Source: CAD feature listing. Evaluate the final solid. Frame: model axes, mm. A direction names the side the tool comes from. Coordinates: 2 decimals unless noted, no trailing zeros. Order: outer loops, then holes, each group sorted by start corner. A loop starts at its lowest first (then second) coordinate and runs counter-clockwise, first axis right, second up. Notation, with made-up numbers: (40.25, 36) -> (96.25, 36) arc R27 cw to (96.25, 65) -> close; hole circle Ø4 at (49, -34). An arc over 180 degrees is marked (long way). Put each result on its own line as item: value.
from build123d import *

# Parameters (mm, degrees)
EXTRUDE_1_DEPTH                   = 3
SKETCH_2_R                        = 1.5
SKETCH_2_R_2                      = 0.75
EXTRUDE_2_DEPTH                   = 73
SKETCH_3_W                        = 42
SKETCH_3_H                        = 3.5
SKETCH_3_W_2                      = 3.2
SKETCH_3_H_2                      = 20.2
CUT_EXTRUDE_1_DEPTH               = 83.725086884
CUT_EXTRUDE_2_REACH               = 84.028
CUT_EXTRUDE_2_OFFSET_FROM_SURFACE = 1.5
CUT_EXTRUDE_START                 = -1.5
SKETCH_4_W                        = 44.5
SKETCH_4_H                        = 1
SKETCH_4_3_W                      = 22
SKETCH_4_3_H                      = 1
CUT_EXTRUDE_3_DEPTH               = 37.5
SKETCH_5_W                        = 3
SKETCH_5_H                        = 1
EXTRUDE_3_DEPTH                   = 34.5
SKETCH_6_R                        = 0.35
CUT_EXTRUDE_4_DEPTH               = 80.653562381
SKETCH_7_W                        = 24.036657481
SKETCH_7_H                        = 1
CUT_EXTRUDE_5_DEPTH               = 1.5
CUT_EXTRUDE_6_DEPTH               = 80.653562381


with BuildPart() as part:
    # 草图1 → 凸台-拉伸1 (new body)
    with BuildSketch(Plane(origin=(0, 0, 0), x_dir=(1, 0, 0), z_dir=(0, 1, 0))):
        Polygon((0, 0), (0, -73), (38.8, -73), (38.8, -47.5), (24.5, 0), align=None)
    extrude(amount=EXTRUDE_1_DEPTH)

    # 草图2 → 凸台-拉伸2 (add)
    # profile 1 of 2: a face of its own
    with BuildSketch(Plane(origin=(0, 0, 0), x_dir=(-1, 0, 0), z_dir=(0, 0, -1))):
        with BuildLine():
            Line((0, 3), (0, 0))
            Line((0, 0), (1.7, 0))
            ThreePointArc((1.7, 0), (0.2, 1.5), (1.7, 3))
            Line((1.7, 3), (0, 3))
        make_face()
    # profile 2 of 2: a face of its own
    with BuildSketch(Plane(origin=(0, 0, 0), x_dir=(-1, 0, 0), z_dir=(0, 0, -1))):
        with Locations((1.7, 1.5)):
            Circle(SKETCH_2_R)
        with Locations((1.7, 1.5)):
            Circle(SKETCH_2_R_2, mode=Mode.SUBTRACT)
    extrude(amount=-EXTRUDE_2_DEPTH)

    # 草图3 → 切除-拉伸1 (cut, through all)
    with BuildSketch(Plane(origin=(0, 3, 0), x_dir=(1, 0, 0), z_dir=(0, 1, 0))):
        with Locations((17.8, -71.25)):
            Rectangle(SKETCH_3_W, SKETCH_3_H)
        with Locations((-1.6, -38.1)):
            Rectangle(SKETCH_3_W_2, SKETCH_3_H_2)
        Polygon((1.3, -3), (22.270157068, -3), (35.8, -47.941785964), (35.8, -69.5), (1.3, -69.5), align=None)
    extrude(amount=-CUT_EXTRUDE_1_DEPTH, mode=Mode.SUBTRACT)

    # 切除-拉伸2: up to this face of the body (flat: up to its plane, moved by the offset)
    cut_extrude_2_end = Plane(part.part.faces().sort_by_distance((29.035078534, 1.5, 25.470892982))[0]).offset(-CUT_EXTRUDE_2_OFFSET_FROM_SURFACE)
    # 草图4 → 切除-拉伸2 (cut, up to the picked face)
    with BuildSketch(Plane(origin=(1.3, 0, 0), x_dir=(0, 0, -1), z_dir=(1, 0, 0)).offset(CUT_EXTRUDE_START), mode=Mode.PRIVATE) as cut_extrude_2_sk1:
        with Locations((-25.25, 1.5)):
            Rectangle(SKETCH_4_W, SKETCH_4_H)
    cut_extrude_2_tool1 = split(extrude(cut_extrude_2_sk1.sketch, amount=CUT_EXTRUDE_2_REACH, mode=Mode.PRIVATE), bisect_by=cut_extrude_2_end, keep=Keep.BOTH, mode=Mode.PRIVATE)
    add(cut_extrude_2_tool1.solids().sort_by(Axis((-0.2, 1.5, 25.25), (1, 0, 0)))[0], mode=Mode.SUBTRACT)

    # 草图4<3> → 切除-拉伸3 (cut)
    with BuildSketch(Plane(origin=(1.3, 0, 0), x_dir=(0, 0, -1), z_dir=(1, 0, 0)).offset(CUT_EXTRUDE_START)):
        with Locations((-58.5, 1.5)):
            Rectangle(SKETCH_4_3_W, SKETCH_4_3_H)
    extrude(amount=CUT_EXTRUDE_3_DEPTH, mode=Mode.SUBTRACT)

    # 草图5 → 凸台-拉伸3 (add)
    with BuildSketch(Plane.ZY.offset(-35.8)):
        with Locations((49.441785964, 2.5)):
            Rectangle(SKETCH_5_W, SKETCH_5_H)
    extrude(amount=EXTRUDE_3_DEPTH)

    # 草图6 → 切除-拉伸4 (cut, through all)
    with BuildSketch(Plane(origin=(0, 3, 0), x_dir=(1, 0, 0), z_dir=(0, 1, 0))):
        with Locations(Location((32.8, -49.441785964, 0), (0, 0, 270))):
            Circle(SKETCH_6_R)
        with Locations(Location((24.9, -49.441785964, 0), (0, 0, 270))):
            Circle(SKETCH_6_R)
    extrude(amount=-CUT_EXTRUDE_4_DEPTH, mode=Mode.SUBTRACT)

    # 草图7 → 切除-拉伸5 (cut)
    with BuildSketch(Plane.XY.offset(3)):
        with Locations((11.818328741, 1.5)):
            Rectangle(SKETCH_7_W, SKETCH_7_H)
    extrude(amount=-CUT_EXTRUDE_5_DEPTH, mode=Mode.SUBTRACT)

    # 草图8 → 切除-拉伸6 (cut, through all)
    with BuildSketch(Plane(origin=(0, 3, 0), x_dir=(1, 0, 0), z_dir=(0, 1, 0))):
        Polygon((20.332372981, 3.436695391), (35.8, -47.941785964), (35.8, -72.849501568), (56.307983414, -72.849501568), (56.307983414, 3.436695391), align=None)
    extrude(amount=-CUT_EXTRUDE_6_DEPTH, mode=Mode.SUBTRACT)


solid = part.part
1. Cut plane B-B on x = 3. Output: boundary loops of the cut face in (y, z), plus the area to 3 significant figures.
Numbers:
outline: (0, 0) -> (3, 0) -> (3, 3) -> (2, 3) -> (2, 1.5) -> (1, 1.5) -> (1, 3) -> (0, 3) -> close; (2, 47.94) -> (3, 47.94) -> (3, 50.94) -> (2, 50.94) -> close
area: 10.5 mm2
2. Cut plane C-C on z = 62. Output: boundary loops of the cut face in (x, y), plus the area to 3 significant figures.
Numbers:
outline: (-1.7, 0) -> (1.3, 0) -> (1.3, 1) -> (-0.2, 1) -> (-0.2, 2) -> (1.3, 2) -> (1.3, 3) -> (-1.7, 3) arc R1.5 ccw to start; hole circle Ø1.5 at (-1.7, 1.5)
area: 9.27 mm2
3. Ray query, line 1 along Z through (x, y) = (8, 2.8); line 2 along Z through (x, y) = (32.8, 2.35); line 3 along X through (y, z) = (2.8, 56). Return the intervals inside material, ascending.
Numbers:
line 1: z = 0 to 3, 47.94 to 50.94
line 2: z = 47.94 to 49.09, 49.79 to 50.94
line 3: x = -2.45 to 1.3
4. Cut plane A-A on z = 34. Output: boundary loops of the cut face in (x, y), plus the area to 3 significant figures.
Numbers:
outline: (0, 0) -> (1.3, 0) -> (1.3, 1) -> (0, 1) -> close; (0, 2) -> (1.3, 2) -> (1.3, 3) -> (0, 3) -> close
area: 2.60 mm2
5. Set-up query: faces 5 (the flat face through (-0.9, 0.9, 48.2)), 6 (the flat face through (1, 2, 33)), 7 (the cylindrical face through (-3.2, 1.5, 58.7)). Return all of +Z, -Z, +X, -X, +Y, -Y with unobstructed straight access to the full face (end or side cutting, diameter ignored); none if empty.
Numbers:
face 5: -X, +Y, -Y
face 6: +Z, +X
face 7: +Z, -Z, -X
6. Cut plane D-D on x = 23.5. Output: boundary loops of the cut face in (y, z).
Numbers:
outline: (2, 47.94) -> (3, 47.94) -> (3, 50.94) -> (2, 50.94) -> close
7. Pull-direction query (Y, two-part tool) for faces 1 (the cylindrical face through (-3.2, 1.5, 13.8)), 2 (the flat face through (9, 2, 0)), 3 (the cylindrical face through (-1.537, 0.768, 13.804)), 4 (the flat face through (1, 1, 26)); classes: pulls with the +Y half, pulls with the -Y half, needs draft (parallel to the pull), parting line crosses it, or undercut.
Numbers:
face 1: parting line crosses it
face 2: needs draft
face 3: undercut
face 4: undercut
8. First-contact query: pin 1 (1.1 mm diameter, centred on y = 0.5, z = 35, fed in from -X); pin 2 (0.5 mm diameter, centred on y = 1.5, z = 11, fed in from +X); pin 3 (0.8 mm diameter, centred on x = 12.5, y = 0.5, fed in from +Z). Flat tips, straight axial feed; report the tip coordinate or a pass-through.
Numbers:
pin 1: stops at x = 0
pin 2: stops at x = -0.2
pin 3: stops at z = 3
